Geometry: see drawing. Coordinates: mm, zero at the bounding-box minimum. A direction names the side the tool comes from. Coordinates: 2 decimals unless noted, no trailing zeros. Loops run counter-clockwise (first coordinate to the right, second up) from the corner with the lowest first, then second, coordinate; pieces in that order, holes last. Notation, with made-up numbers: (49.25, 21) -> (80.25, 21) arc R16 ccw to (80.25, 45) -> close; hole circle Ø11 at (25.25, 61.25). An arc over 180 degrees is marked (long way). Answer as a JSON object with one key per item and string values.
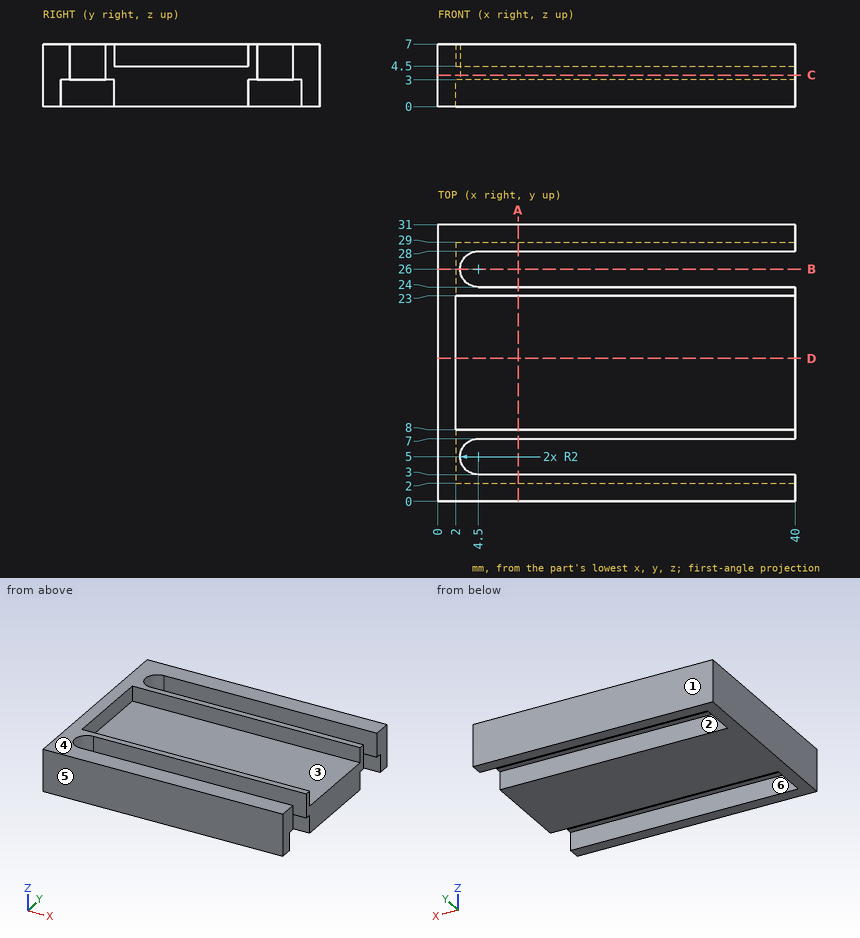
1. Mould query, pull axis Y, two halves, no side actions, for the marked faces 3, 4, 5 and 6. Classes: pulls with the +Y half, pulls with the -Y half, needs draft (parallel to the pull), parting line crosses it, or undercut.
Reply:
{"face 3": "undercut", "face 4": "needs draft", "face 5": "pulls with the -Y half", "face 6": "undercut"}
2. Section query A-A (x = 9). Return loops of the section in (y, z).
Reply:
{"outline": "(0, 0) -> (2, 0) -> (2, 3) -> (3, 3) -> (3, 7) -> (0, 7) -> close; (7, 3) -> (8, 3) -> (8, 0) -> (23, 0) -> (23, 3) -> (24, 3) -> (24, 7) -> (23, 7) -> (23, 4.5) -> (8, 4.5) -> (8, 7) -> (7, 7) -> close; (28, 3) -> (29, 3) -> (29, 0) -> (31, 0) -> (31, 7) -> (28, 7) -> close"}
3. Section query D-D (y = 16). Return loops of the section in (x, z).
Reply:
{"outline": "(0, 0) -> (40, 0) -> (40, 4.5) -> (2, 4.5) -> (2, 7) -> (0, 7) -> close"}
4. Section query C-C (z = 3.5). Return loops of the section in (x, y).
Reply:
{"outline": "(0, 0) -> (40, 0) -> (40, 3) -> (4.5, 3) arc R2 cw to (4.5, 7) -> (40, 7) -> (40, 24) -> (4.5, 24) arc R2 cw to (4.5, 28) -> (40, 28) -> (40, 31) -> (0, 31) -> close"}
5. Section query B-B (y = 26). Return loops of the section in (x, z), plus the area to 3 significant figures.
Reply:
{"outline": "(0, 0) -> (2, 0) -> (2, 3) -> (2.5, 3) -> (2.5, 7) -> (0, 7) -> close", "area": "16.0 mm2"}
6. Pin query (flat end, axial travel): P1, Ø1.5, axis at y = 4, z = 2, coming from the +X side; P2, Ø8, axis at x = 31, y = 9, coming from the +Z side; P3, Ø4.5, axis at x = 23.5, y = 15, coming from the +Z side. Return the tip coordinate at first contact, or that it passes through.
Reply:
{"P1": "stops at x = 2", "P2": "stops at z = 7", "P3": "stops at z = 4.5"}
7. Access query for the marked faces 1 and 2. Directions: +Z, -Z, +X, -X, +Y, -Y. A direction counts if a zero-diameter tool reaches every point of the face in a straight line with its end or side. Return the directions, or none.
Reply:
{"face 1": "+Z, -Z, +X, -X, +Y", "face 2": "-Z, +X"}
8. Line query: line 1 along Y through (x, z) = (4, 1); line 2 along Y through (x, z) = (17.5, 4.75); line 3 along Y through (x, z) = (19, 3.5). Output: solid intervals per line, ascending.
Reply:
{"line 1": "y = 0 to 2, 8 to 23, 29 to 31", "line 2": "y = 0 to 3, 7 to 8, 23 to 24, 28 to 31", "line 3": "y = 0 to 3, 7 to 24, 28 to 31"}
